For this review, take the finished solid that the model builds, in its own axes (mm). Face numbers are marked on the shaded views. Round coordinates to 2 decimals unless told otherwise and drop trailing zeros. Loops run counter-clockwise (first coordinate to the right, second up) from the corner with the lowest first, then second, coordinate; pieces in that order, holes last.
1. Consider section A-A on z = 10.5. State the section outline as (x, y) points.
2. Consider section B-B on y = 0. State the section outline as (x, z) points.
3. Draft analysis for pull direction Y (two halves, no side actions). For the marked faces 1, 2, 3 and 4, state which applies: released by +Y, released by -Y, zero draft, split by the parting line, or undercut.
4. Clearance check with flat-ended pins moving along their axes: pin 1 Ø1.5 at (x, y) = (1.5, -20) entering from -Z; pin 2 Ø3.5 at (x, y) = (-5.5, -25.5) entering from -Z; pin 3 Ø2.5 at (x, y) = (4.5, 10.5) entering from -Z; pin 4 Ø10 at (x, y) = (0, -2.5) entering from -Z. State where each tip first meets the part, or that it passes through.
5. Consider section C-C on z = 37. State the section outline as (x, y) points, then the cut area to 3 significant figures.
6. To check wall thickness, follow line 1 along Y through (x, z) = (0, 58.25); line 2 along Z through (x, y) = (1, 12.5); line 3 along Z through (x, y) = (-4.75, 1). State the ranges of each line that lie inside material, in increasing order.
7. Consider section D-D on z = 60. State the section outline as (x, y) points, then the cut area to 3 significant figures.
from build123d import *

# Parameters (mm, degrees)
SKETCH_W        = 24
SKETCH_H        = 78
PAD_DEPTH       = 70
SKETCH001_R     = 8.5
POCKET_DEPTH    = 30
POCKET001_DEPTH = 70
POCKET002_DEPTH = 24


with BuildPart() as part:
    # Sketch → Pad (new body)
    with BuildSketch(Plane.XY):
        Rectangle(SKETCH_W, SKETCH_H)
    extrude(amount=PAD_DEPTH)

    # Sketch001 (on Face6 of Pad) → Pocket (cut)
    with BuildSketch(Plane.XY.offset(70)):
        Circle(SKETCH001_R)
    extrude(amount=-POCKET_DEPTH, mode=Mode.SUBTRACT)

    # Sketch002 (on Face5 of Pocket) → Pocket001 (cut)
    with BuildSketch(Plane.XY.offset(70)):
        with BuildLine():
            ThreePointArc((-10.723805, 39), (0, 34), (10.723805, 39))
            Line((-10.723805, 39), (10.723805, 39))
        make_face()
        with BuildLine():
            ThreePointArc((10.723805, -39), (0, -34), (-10.723805, -39))
            Line((-10.723805, -39), (10.723805, -39))
        make_face()
    extrude(amount=-POCKET001_DEPTH, mode=Mode.SUBTRACT)

    # Sketch003 (on Face9 of Pocket001) → Pocket002 (cut)
    with BuildSketch(Plane.YZ.offset(12)):
        Polygon((-27, 3), (-27, 0), (27, 0), (27, 3), (24, 3), (24, 6), (21, 6), (21, 9), (18, 9), (18, 12), (15, 12), (15, 15), (12, 15), (12, 18), (9, 18), (9, 21), (6, 21), (6, 24), (3, 24), (3, 27), (-3, 27), (-3, 24), (-6, 24), (-6, 21), (-9, 21), (-9, 18), (-12, 18), (-12, 15), (-15, 15), (-15, 12), (-18, 12), (-18, 9), (-21, 9), (-21, 6), (-24, 6), (-24, 3), align=None)
    extrude(amount=-POCKET002_DEPTH, mode=Mode.SUBTRACT)


solid = part.part
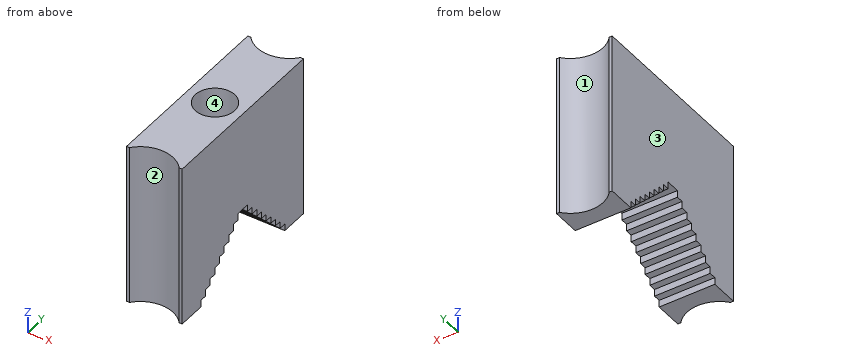
Resolved:
1. outline: (-12, -39) - (-10.72, -39) arc R14 cw to (10.72, -39) - (12, -39) - (12, -18) - (-12, -18) - close; (-12, 18) - (12, 18) - (12, 39) - (10.72, 39) arc R14 cw to (-10.72, 39) - (-12, 39) - close
2. outline: (-12, 27) - (12, 27) - (12, 70) - (8.5, 70) - (8.5, 40) - (-8.5, 40) - (-8.5, 70) - (-12, 70) - close
3. face 1: released by +Y
3. face 2: released by -Y
3. face 3: zero draft
3. face 4: undercut
4. pin 1: stops at z = 9
4. pin 2: stops at z = 0
4. pin 3: stops at z = 18
4. pin 4: stops at z = 21
5. outline: (-12, -39) - (-10.72, -39) arc R14 cw to (10.72, -39) - (12, -39) - (12, 39) - (10.72, 39) arc R14 cw to (-10.72, 39) - (-12, 39) - close
5. area: 1,720 mm2
6. line 1: y = -34 to -8.5, 8.5 to 34
6. line 2: z = 15 to 70
6. line 3: z = 27 to 40
7. outline: (-12, -39) - (-10.72, -39) arc R14 cw to (10.72, -39) - (12, -39) - (12, 39) - (10.72, 39) arc R14 cw to (-10.72, 39) - (-12, 39) - close; hole circle Ø17 at (0, 0)
7. area: 1,500 mm2
